Geometry check sheet. Reference: drawing and pictorial views, mm from the part's lowest x, y, z. Give positions to 0.01 mm unless a question says otherwise; leave off trailing zeros. Loops run counter-clockwise (first coordinate to the right, second up) from the corner with the lowest first, then second, coordinate; pieces in that order, holes last. Notation, with made-up numbers: (88, 55.25) - (147, 55.25) arc R32 ccw to (147, 91.25) - close; hole circle Ø2 at (-20, -23.5). An arc over 180 degrees is marked (long way). Use CSV: the item, a comma, the result in double quotes.
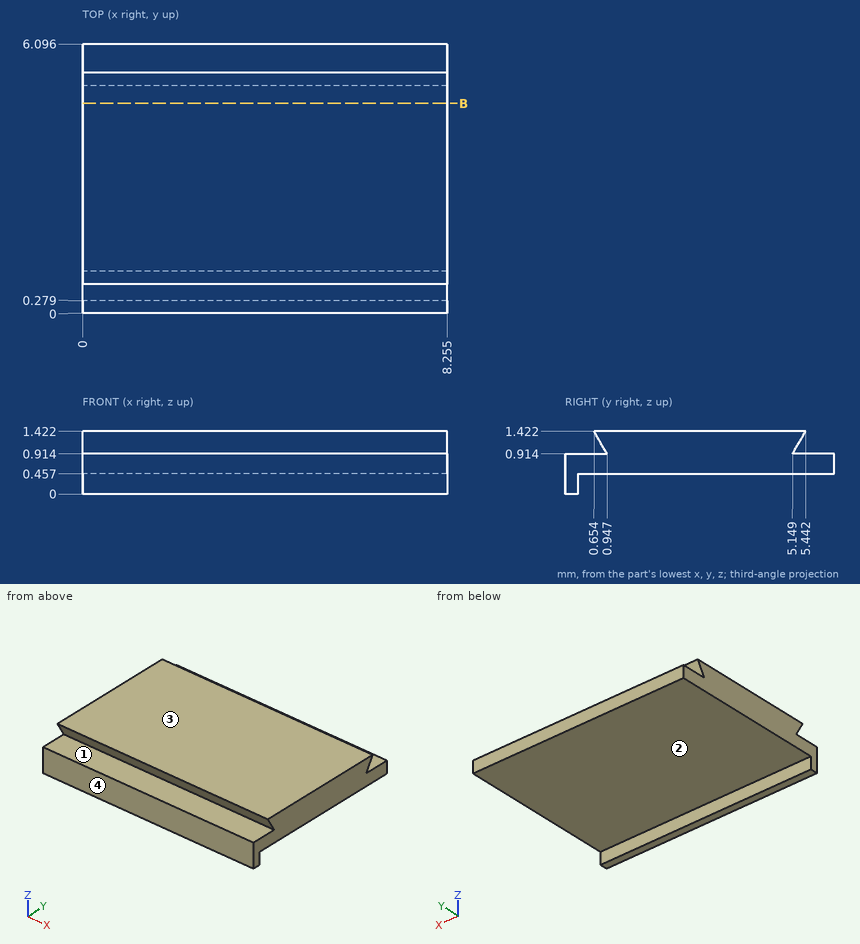
1. Scan lines: line 1 along Z through (x, y) = (1.5, 3); line 2 along Z through (x, y) = (6.5, 0.5) (1 decimal); line 3 along Y through (x, z) = (2.75, 0.1). Record each from-to range of solid material in increasing order.
Completed:
line 1,"z = 0.46 to 1.42"
line 2,"z = 0.5 to 0.9"
line 3,"y = 0 to 0.28"
2. Go/stop test with flat-tipped pins: pin 1 Ø1.7 at (x, y) = (3, 4) entering from -Z; pin 2 Ø0.5 at (x, y) = (4, 6) entering from +Z. Record where each tip stops, or that it passes through.
Completed:
pin 1,"stops at z = 0.46"
pin 2,"stops at z = 0.91"
3. Sectioned sample at B-B, the plane y = 4.75. Record the boundary of the cut face in (x, z) (1 decimal).
Completed:
outline,"(0, 0.5) - (8.3, 0.5) - (8.3, 1.4) - (0, 1.4) - close"
4. Release check for a two-part mould opening along Z. For the marked faces 1, 2, 3 and 4 record: released by +Z, released by -Z, zero draft, split by the parting line, or undercut.
Completed:
face 1,"undercut"
face 2,"released by -Z"
face 3,"released by +Z"
face 4,"zero draft"
